Build history of the part. All positions in model axes, mm. A direction names the side the tool comes from. Coordinates: 2 decimals unless noted, no trailing zeros. Loops run counter-clockwise (first coordinate to the right, second up) from the corner with the lowest first, then second, coordinate; pieces in that order, holes last.
Item 1: Cut at B-B (x = 0). List the corners of the cut face in (y, z), and give its area (3 significant figures).
Item 2: Drill centre lines: line 1 along Z through (x, y) = (0, 2.85); line 2 along Y through (x, z) = (1.5, 2.2); line 3 along Y through (x, z) = (-1, 0.75). Where is each one in solid material? Low to high.
Item 3: Cut at C-C (y = 4.25). List the corners of the cut face in (x, z).
Item 4: Flat gauge pin, fed straight in: pin 1 (0.9 mm diameter, centred on x = -0.5, z = 0, fed in from -Y). Where does the tip first touch, or does it go through?
Item 5: Cut at A-A (y = 1.75). List the corners of the cut face in (x, z), and give its area (3 significant figures).
Item 6: Cut at D-D (z = 0.65). List the corners of the cut face in (x, y).
Item 7: 3-axis set-ups, long thin cutter, end or side, ignore diameter. For faces 5 (the face through (-1.5, 8.96, -0.07)), 6 (the face through (0, 4, 0)), 7 (the face through (-2.39, 2.96, 1.36)): which of +Z, -Z, +X, -X, +Y, -Y reach the whole face in a straight line?
Item 8: Mould opens along Z. For faces 1 (the face through (1.4, 6, -1.3)), 2 (the face through (-1.5, 1.97, 0.07)), 3 (the face through (2.37, 2.958, 1.394)), 4 (the face through (2.39, 2.96, -1.36)) say: released by +Z, released by -Z, zero draft, split by the parting line, or undercut.
from build123d import *

# Parameters (mm, degrees)
EXTRUDE_1_DEPTH     = 6
SKETCH_2_R          = 1.5
CUT_EXTRUDE_1_DEPTH = 4
SKETCH_3_R          = 1.5
EXTRUDE_2_DEPTH     = 6


with BuildPart() as part:
    # 草图1 → 凸台-拉伸1 (new body)
    with BuildSketch(Plane(origin=(0, 0, 0), x_dir=(1, 0, 0), z_dir=(0, 1, 0))):
        Polygon((3.175426481, 0), (1.58771324, 2.75), (-1.58771324, 2.75), (-3.175426481, 0), (-1.58771324, -2.75), (1.58771324, -2.75), align=None)
    extrude(amount=EXTRUDE_1_DEPTH)

    # 草图2 → 切除-拉伸1 (cut)
    with BuildSketch(Plane.XZ):
        Circle(SKETCH_2_R)
    extrude(amount=-CUT_EXTRUDE_1_DEPTH, mode=Mode.SUBTRACT)

    # 草图3 → 凸台-拉伸2 (add)
    with BuildSketch(Plane(origin=(0, 6, 0), x_dir=(1, 0, 0), z_dir=(0, 1, 0))):
        Circle(SKETCH_3_R)
    extrude(amount=EXTRUDE_2_DEPTH)


solid = part.part
Filled sheet:
1. outline: (0, -2.75) - (6, -2.75) - (6, -1.5) - (12, -1.5) - (12, 1.5) - (6, 1.5) - (6, 2.75) - (0, 2.75) - (0, 1.5) - (4, 1.5) - (4, -1.5) - (0, -1.5) - close
1. area: 39.0 mm2
2. line 1: z = -2.75 to -1.5, 1.5 to 2.75
2. line 2: y = 0 to 6
2. line 3: y = 4 to 12
3. outline: (-3.18, 0) - (-1.59, -2.75) - (1.59, -2.75) - (3.18, 0) - (1.59, 2.75) - (-1.59, 2.75) - close
4. pin 1: stops at y = 4
5. outline: (-3.18, 0) - (-1.59, -2.75) - (1.59, -2.75) - (3.18, 0) - (1.59, 2.75) - (-1.59, 2.75) - close; hole circle Ø3 at (0, 0)
5. area: 19.1 mm2
6. outline: (-2.8, 0) - (-1.35, 0) - (-1.35, 4) - (1.35, 4) - (1.35, 0) - (2.8, 0) - (2.8, 6) - (1.35, 6) - (1.35, 12) - (-1.35, 12) - (-1.35, 6) - (-2.8, 6) - close
7. face 5: +Y
7. face 6: -Y
7. face 7: +Z, -X, +Y, -Y
8. face 1: zero draft
8. face 2: undercut
8. face 3: released by +Z
8. face 4: released by -Z
